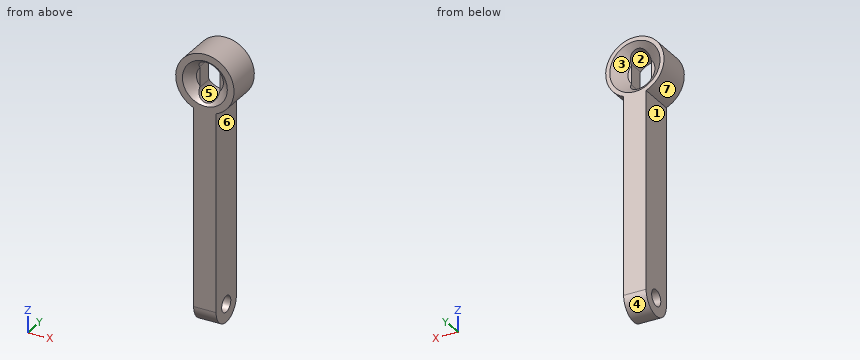
```python
from build123d import *

# Parameters (mm, degrees)
SKETCH1_R      = 3.25
EXTRUDE1_DEPTH = 4
SKETCH2_R      = 0.9
EXTRUDE2_DEPTH = 1.25


with BuildPart() as part:
    # Sketch1 → Extrude1 (new body)
    with BuildSketch(Plane(origin=(0, 0, 0), x_dir=(1, 0, 0), z_dir=(0, 1, 0))):
        with Locations(Location((0, 0, 0), (0, 0, 270))):  # turned: the seam where the file's is
            Circle(SKETCH1_R)
        with BuildLine():
            Line((1.1, 1.15), (1.1, -1.15))
            ThreePointArc((1.1, -1.15), (0, -2.25), (-1.1, -1.15))
            Line((-1.1, -1.15), (-1.1, 1.15))
            ThreePointArc((-1.1, 1.15), (0, 2.25), (1.1, 1.15))
        make_face(mode=Mode.SUBTRACT)
    extrude(amount=EXTRUDE1_DEPTH)

    # Sketch2 → Extrude2 (add, symmetric)
    with BuildSketch(Plane(origin=(0, 0, 0), x_dir=(0, 0, -1), z_dir=(1, 0, 0))):
        with BuildLine():
            Line((3, 4), (3, 0))
            Line((3, 0), (25, 0))
            ThreePointArc((25, 0), (27, 2), (25, 4))
            Line((25, 4), (3, 4))
        make_face()
        with Locations((25, 2)):
            Circle(SKETCH2_R, mode=Mode.SUBTRACT)
    extrude(amount=EXTRUDE2_DEPTH, both=True)

    # Sketch4 → Cut-Revolve1 (revolve, cut)
    with BuildSketch(Plane(origin=(0, 0, 0), x_dir=(0, 0, -1), z_dir=(1, 0, 0))):
        Polygon((0, 2.7), (1.5, 2.7), (2.8, 4), (0, 4), align=None)
        Polygon((0, 1), (1.5, 1), (2.5, 0), (0, 0), align=None)
    revolve(axis=Axis((0, 0, 0), (0, 1, 0)), mode=Mode.SUBTRACT)


solid = part.part
```
Could you check a few things on this model? Use its own coordinates, in mm. Face numbers are marked on the shaded views. A direction names the side the tool comes from. Round coordinates to 2 decimals unless told otherwise and drop trailing zeros. Loops run counter-clockwise (first coordinate to the right, second up) from the corner with the lowest first, then second, coordinate; pieces in that order, holes last. Notation, with made-up numbers: M 41.25,53 L 71.25,53 A30 ccw 71.25,86 Z; hole C -31,8 d6. An arc over 180 degrees is marked long. Put each result on its own line as item: value.
Q1. Imagine slicing it at C-C (x = 0.25). State how many separate pieces and enclosed holes the cut face has, then the cut area to 3 significant figures.
Check result:
separate pieces: 2
enclosed holes: 1
area: 98.5 mm2
Q2. On a 3-axis mill with a long thin cutter (end or side, diameter ignored), from which of +Z, -Z, +X, -X, +Y, -Y can I reach the whole of each face in a straight line? I mean the marked faces 1, 2 and 3. Say none if no direction works.
Check result:
face 1: -Z, -X, +Y, -Y
face 2: +Y, -Y
face 3: +Y
Q3. I need wall thicknesses on probe 1 along Y at (x, z) = (-0.05, -25); probe 2 along X at (y, z) = (0.6, -4); probe 3 along Z at (x, y) = (-1, 1.4). Which ranges of each line are inside material? Lowest first, please.
Check result:
probe 1: 0 to 1.1, 2.9 to 4
probe 2: -1.25 to 1.25
probe 3: -26.91 to -25.67, -24.33 to -1.61, 1.61 to 3.09
Q4. Imagine slicing it at A-A (z = 0). Write out the boundary of the cut face in (x, y), then the cut area to 3 significant figures.
Check result:
outline: M -3.25,0 L -2.5,0 L -1.5,1 L -1.1,1 L -1.1,2.7 L -1.5,2.7 L -2.8,4 L -3.25,4 Z; M 1.1,1 L 1.5,1 L 2.5,0 L 3.25,0 L 3.25,4 L 2.8,4 L 1.5,2.7 L 1.1,2.7 Z
area: 12.7 mm2
Q5. Imagine slicing it at D-D (z = -8.5). Write out the boundary of the cut face in (x, y).
Check result:
outline: M -1.25,0 L 1.25,0 L 1.25,4 L -1.25,4 Z
Q6. Thinking about a two-plate mould opening in Z: for the marked faces 4, 5, 6 and 7, which applies, released by +Z, released by -Z, zero draft, split by the parting line, or undercut?
Check result:
face 4: released by -Z
face 5: undercut
face 6: zero draft
face 7: split by the parting line
Q7. For pin 1 (2 mm diameter, centred on y = 2.5, z = -11.5, fed in from +X); pin 2 (2 mm diameter, centred on y = 3, z = -8.5, fed in from -X), each with a flat end and sliding along its axis, tell me the tip position at first contact or that it passes through.
Check result:
pin 1: x = 1.25
pin 2: x = -1.25
Q8. Imagine slicing it at B-B (y = 2). Write out the boundary of the cut face in (x, z).
Check result:
outline: M -1.25,-27 L 1.25,-27 L 1.25,-25.9 L -1.25,-25.9 Z; M -1.25,-24.1 L 1.25,-24.1 L 1.25,-3 A3.25 ccw long -1.25,-3 Z; hole M -1.1,-1.15 A1.1 ccw 1.1,-1.15 L 1.1,1.15 A1.1 ccw -1.1,1.15 Z
